Source: CAD feature listing. Evaluate the final solid. Frame: model axes, mm. A direction names the side the tool comes from. Round coordinates to 2 decimals unless told otherwise and drop trailing zeros. Order: outer loops, then holes, each group sorted by start corner. A loop starts at its lowest first (then second) coordinate and runs counter-clockwise, first axis right, second up. Notation, with made-up numbers: (11, -23.5) - (33, -23.5) arc R23 ccw to (33, 4.5) - close; hole circle Ø7 at (-18.5, 83.5). An arc over 180 degrees is marked (long way). Return JSON: item names as keys, results as strings. Group by question number.
1) Access query for faces 1 (the flat face through (-2.7, 13, 1.5)), 2 (the flat face through (-2.7, 12.5, 0.5)), 3 (the flat face through (-2.7, -13, 1.5)). Directions: +Z, -Z, +X, -X, +Y, -Y. A direction counts if a zero-diameter tool reaches every point of the face in a straight line with its end or side. Return the directions, or none.
2) Contact query for flat-ended pins moving along their axis: P1, Ø10, axis at x = 11.5, y = 3, coming from the -Z side; P2, Ø0.8, axis at x = 0.5, z = 2.5, coming from the +Y side; P3, Ø0.5, axis at x = 4, z = 1.5, coming from the +Y side; P4, Ø0.9, axis at y = -13.5, z = 1.5, coming from the -X side. Output: stop coordinate, or through.
3) Section A-A, the plane x = -19. Return loops of the section in (y, z), plus the area to 3 significant figures.
4) Ray query, line 1 (Y direction, x = -5, z = 1.7); line 2 (Y direction, x = -17.5, z = 0.8). Return the intervals inside material, ascending. Write a range as from..to.
5) Mould query, pull axis Z, two halves, no side actions, for faces 4 (the flat face through (-1, 0, 0)), 5 (the flat face through (-2.7, 12.5, 2.5)), 6 (the flat face through (-1, 0, 3)). Classes: pulls with the +Z half, pulls with the -Z half, needs draft (parallel to the pull), parting line crosses it, or undercut.
```python
from build123d import *

# Parameters (mm, degrees)
SKETCH1_W           = 45
SKETCH1_H           = 25
BOSS_EXTRUDE1_DEPTH = 3
SKETCH2_W           = 3
SKETCH2_H           = 3
BOSS_EXTRUDE2_DEPTH = 3
SKETCH3_W           = 1
SKETCH3_H           = 0.5
BOSS_EXTRUDE3_DEPTH = 45
SKETCH4_W           = 3
SKETCH4_H           = 25
BOSS_EXTRUDE4_DEPTH = 3
FILLET1_R           = 3


with BuildPart() as part:
    # Sketch1 → Boss-Extrude1 (new body)
    with BuildSketch(Plane.XY):
        Rectangle(SKETCH1_W, SKETCH1_H)
    extrude(amount=BOSS_EXTRUDE1_DEPTH)

    # Sketch2 → Boss-Extrude2 (add)
    with BuildSketch(Plane(origin=(22.5, 0, 0), x_dir=(0, 0, -1), z_dir=(1, 0, 0))):
        with Locations((-1.5, -14)):
            Rectangle(SKETCH2_W, SKETCH2_H)
        with Locations((-1.5, 14)):
            Rectangle(SKETCH2_W, SKETCH2_H)
    extrude(amount=-BOSS_EXTRUDE2_DEPTH)

    # Sketch3 → Boss-Extrude3 (add)
    with BuildSketch(Plane.ZY.offset(-19.5)):
        with Locations((1.5, -12.75)):
            Rectangle(SKETCH3_W, SKETCH3_H)
        with Locations((1.5, 12.75)):
            Rectangle(SKETCH3_W, SKETCH3_H)
    extrude(amount=BOSS_EXTRUDE3_DEPTH)

    # Sketch4 → Boss-Extrude4 (add)
    with BuildSketch(Plane.ZY.offset(22.5)):
        with Locations((1.5, 0)):
            Rectangle(SKETCH4_W, SKETCH4_H)
    extrude(amount=BOSS_EXTRUDE4_DEPTH)

    # Fillet1
    fillet1_edges = [part.edges().sort_by_distance(p)[0] for p in [
        (22.5, 15.5, 1.5),
        (22.5, -15.5, 1.5),
    ]]
    fillet(fillet1_edges, radius=FILLET1_R - 0.0001)  # a hair under: the kernel refuses the full size


solid = part.part
```
Geometry check:
{
 "1": {"face 1": "+Z, -Z, -X, +Y", "face 2": "-Z, -X, +Y", "face 3": "+Z, -Z, -X, -Y"},
 "2": {"P1": "z = 0", "P2": "y = 12.5", "P3": "y = 13", "P4": "x = 19.5"},
 "3": {"outline": "(-13, 1) - (-12.5, 1) - (-12.5, 0) - (12.5, 0) - (12.5, 1) - (13, 1) - (13, 2) - (12.5, 2) - (12.5, 3) - (-12.5, 3) - (-12.5, 2) - (-13, 2) - close", "area": "76.0 mm2"},
 "4": {"line 1": "-13..13", "line 2": "-12.5..12.5"},
 "5": {"face 4": "pulls with the -Z half", "face 5": "needs draft", "face 6": "pulls with the +Z half"}
}
